Autodesk Inventor part; units mm, degrees
ref_plane "Work Plane1" through (0, 0, -15) normal (0, 0, 1) x (1, 0, 0)
ref_plane "YZ Plane" through (0, 0, 0) normal (1, 0, 0) x (0, 1, 0)
ref_plane "XZ Plane" through (0, 0, 0) normal (0, 1, 0) x (-1, 0, 0)
sketch "Sketch1" plane through (0, 0, 0) normal (0, 0, 1) x (1, 0, 0)
  line L0 (0, 0) -> (25, 0)
  line L1 (25, 0) -> (25, 40)
  line L2 (25, 40) -> (0, 40)
  line L3 (0, 40) -> (0, 0)
  dimension "d1" = 25
  dimension "d2" = 40
  dimension "d3" = 25
extrude "Extrusion1" add sketch "Sketch1" against normal blind 30
sketch "Sketch2" plane through (25, 0, 0) normal (1, 0, 0) x (0, 0, -1)
  line L0 (0, 0) -> (30, 0)
  circle A0 centre (15, 6.56) radius 2.46
extrude "Extrusion2" cut sketch "Sketch2" against normal blind 30
sketch "Sketch3" plane through (0, 0, 0) normal (-1, 0, 0) x (0, 0, 1)
  line L0 (0, 0) -> (-30, 0)
  line L1 (-25.05, 0) -> (-4.95, 0)
  line L2 (-4.95, 0) -> (-4.95, 33.12)
  line L3 (-4.95, 33.12) -> (-25.05, 33.12)
  line L4 (-25.05, 33.12) -> (-25.05, 0)
  dimension "d11" = 20.1
extrude "Extrusion3" cut sketch "Sketch3" against normal blind 20
sketch "Sketch4" plane through (0, 0, 0) normal (0, -1, 0) x (1, 0, 0)
  line L0 (20, -4.95) -> (20, -25.05)
  line L1 (20, -15) -> (25, -15)
  line L2 (25, 0) -> (25, -30)
  line L3 (20, -8.025) -> (25, -8.025)
  line L4 (25, -8.025) -> (25, -21.975)
  line L5 (25, -21.975) -> (20, -21.975)
  line L6 (20, -21.975) -> (20, -8.025)
  line L7 (20, -8.025) -> (25, -21.975) construction
  line L8 (25, -8.025) -> (20, -21.975) construction
  line L9 (25, -12.54) -> (25, -17.46)
  point P0 (0, 0)
  point P1 (22.5, -15)
  dimension "d14" = 13.95
extrude "Extrusion4" add sketch "Sketch4" along normal blind 15
sketch "Sketch5" plane through (20, 0, 0) normal (-1, 0, 0) x (0, 0, 1)
  circle A0 centre (-15, 6.56) radius 2.46
  circle A1 centre (-15, 6.56) radius 4.7025
  circle A2 centre (-15, 6.56) radius 2.46
  circle A3 centre (-15, 6.56) radius 2.46
  point P0 (0, 0)
  dimension "d17" = 9.405
extrude "Extrusion5" cut sketch "Sketch5" against normal blind 2.1
sketch "Sketch6" plane through (25, 0, 0) normal (1, 0, 0) x (0, 0, -1)
  circle A0 centre (15, 6.56) radius 4.7025
  line L0 (15, 6.56) -> (15, 23.56)
  circle A1 centre (15, 23.56) radius 2.46
  point P0 (0, 0)
  dimension "d20" = 17
  dimension "d21" = 4.92
extrude "Extrusion6" cut sketch "Sketch6" against normal blind 10 contours A1
sketch "Sketch7" plane through (20, 0, 0) normal (-1, 0, 0) x (0, 0, 1)
  circle A0 centre (-15, 23.56) radius 2.46
  circle A1 centre (-15, 23.56) radius 4.7025
  point P0 (0, 0)
  dimension "d24" = 9.405
extrude "Extrusion7" cut sketch "Sketch7" against normal blind 2.1
sketch "Sketch9" plane through (25, 0, 0) normal (1, 0, 0) x (0, 0, -1)
  circle A0 centre (15, 6.56) radius 2.46
  circle A1 centre (15, 6.56) radius 2.46
  circle A2 centre (15, 23.56) radius 2.46
  circle A3 centre (15, 23.56) radius 2.46
  line L0 (30, 40) -> (30, 0)
  line L1 (30, 0) -> (30, 40)
  line L2 (30, 40) -> (0, 40)
  line L3 (0, 40) -> (0, 0)
  line L4 (0, 0) -> (8.025, 0)
  line L5 (21.975, 0) -> (21.975, -15)
  line L6 (21.975, -15) -> (8.025, -15)
  line L7 (8.025, -15) -> (8.025, 0)
  line L8 (0, 0) -> (8.025, 0)
  line L9 (21.975, 0) -> (30, 0)
extrude "Extrusion8" add sketch "Sketch9" along normal blind 5
sketch "Sketch10" plane through (0, 40, 0) normal (0, 1, 0) x (1, 0, 0)
  line L0 (0, 30) -> (30, 30)
  line L1 (30, 0) -> (0, 0)
  line L2 (0, 30) -> (30, 30)
  line L3 (30, 30) -> (30, 0)
  line L4 (30, 0) -> (0, 0)
  line L5 (0, 0) -> (0, 30)
extrude "Extrusion9" add sketch "Sketch10" along normal blind 30
sketch "Sketch12" plane through (30, 0, 0) normal (1, 0, 0) x (0, 0, -1)
  circle A0 centre (15, 6.56) radius 2.46
  line L0 (15, 6.56) -> (15, 15.06)
  circle A1 centre (15, 15.06) radius 2.525
  point P0 (0, 0)
  dimension "d31" = 8.5
  dimension "d33" = 5.05
extrude "Extrusion10" cut sketch "Sketch12" against normal blind 30 contours A1
sketch "Sketch15" plane through (0, 0, -25.05) normal (-1, 0, 0) x (0, 0, 1)
  line L0 (0, 33.12) -> (20.1, 33.12)
  line L1 (20.1, 33.12) -> (20.1, 0)
  line L2 (0, 33.12) -> (20.1, 33.12)
  line L3 (20.1, 33.12) -> (20.1, 31.1)
  line L4 (20.1, 31.1) -> (0, 31.1)
  line L5 (0, 31.1) -> (0, 33.12)
  point P0 (25.05, 0)
  dimension "d57" = 2.02
extrude "Extrusion13" add sketch "Sketch15" against normal blind 20
sketch "Sketch17" plane through (0, 0, 0) normal (0, 0, 1) x (1, 0, 0)
  line L0 (0, 70) -> (30, 70)
  line L1 (30, 70) -> (50.0622, 90.0622)
  line L2 (30, 70) -> (80, 70) construction
  line L3 (11.9522, 97.2454) -> (0, 85.2932)
  line L4 (0, 70) -> (0, 85.2932)
  line L5 (0, 70) -> (0, 0)
  line L6 (0, 70) -> (30, 70)
  line L7 (10.923, 112.2849) -> (0, 120.567)
  line L8 (50.0622, 105.3553) -> (50.0622, 120.567)
  line L9 (50.0622, 105.3553) -> (50.0622, 90.0622)
  arc A0 (11.9522, 97.2454) -> (10.923, 112.2849) centre (4.8811, 104.3165) ccw
  line L10 (0, 156.567) -> (30, 156.567)
  line L11 (30, 156.567) -> (50.0622, 120.567)
  line L12 (5, 154.567) -> (0, 156.567)
  line L13 (5, 122.567) -> (0, 120.567)
  line L14 (5, 122.567) -> (10, 138.567)
  line L15 (10, 138.567) -> (5, 154.567)
  dimension "d61" = 45
  dimension "d62" = 32.0271
  dimension "d72" = 10
extrude "Extrusion14" add sketch "Sketch17" against normal blind 30
sketch "Sketch23" plane through (0, 0, 0) normal (0, 0, 1) x (1, 0, 0)
  line L0 (50.0622, 90.0622) -> (30, 70)
  line L1 (30, 70) -> (50.0622, 90.0622)
  line L2 (50.0622, 120.567) -> (50.0622, 90.0622)
  line L3 (50.0622, 90.0622) -> (50.0622, 120.567)
  line L4 (30, 156.567) -> (50.0622, 120.567)
  line L5 (50.0622, 120.567) -> (30, 156.567)
  line L6 (0, 156.567) -> (30, 156.567)
  line L7 (30, 156.567) -> (0, 156.567)
  line L8 (5, 154.567) -> (0, 156.567)
  line L9 (0, 156.567) -> (5, 154.567)
  line L10 (10, 138.567) -> (5, 154.567)
  line L11 (5, 154.567) -> (10, 138.567)
  line L12 (5, 122.567) -> (10, 138.567)
  line L13 (10, 138.567) -> (5, 122.567)
  line L14 (0, 120.567) -> (5, 122.567)
  line L15 (5, 122.567) -> (0, 120.567)
  line L16 (10.923, 112.2849) -> (0, 120.567)
  line L17 (0, 120.567) -> (10.923, 112.2849)
  line L18 (0, 85.2932) -> (11.9522, 97.2454)
  line L19 (11.9522, 97.2454) -> (0, 85.2932)
  line L20 (0, 85.2932) -> (0, 55.2932)
  line L21 (0, 0) -> (0, 85.2932)
  line L22 (0, 55.2932) -> (30, 55.2932)
  line L23 (30, 0) -> (30, 70)
  line L24 (30, 55.2932) -> (30, 70)
  arc A0 (11.9522, 97.2454) -> (10.923, 112.2849) centre (4.8811, 104.3165) ccw
  dimension "d97" = 30
extrude "Extrusion15" add sketch "Sketch23" along normal blind 30
ref_plane "Work Plane1" through (0, 0, -15) normal (0, 0, 1) x (1, 0, 0)
mirror "Mirror1" about plane through (0, 0, -15) normal (0, 0, 1) of "Extrusion15"
properties part number "rec_c_32mm_x_90mm"
Here's how the part is built. I have some questions about the finished solid (model axes, mm). A direction names the side the tool comes from. Give positions to 0.01 mm unless a question says otherwise; leave off trailing zeros. Loops run counter-clockwise (first coordinate to the right, second up) from the corner with the lowest first, then second, coordinate; pieces in that order, holes last. Notation, with made-up numbers: (29.5, 72) -> (88.5, 72) arc R21 ccw to (88.5, 86) -> close; hole circle Ø7 at (74.5, -26.75). An arc over 180 degrees is marked (long way). Answer as a JSON object with one key per item and string values. Group by question number.
Item 1: On a 3-axis mill with a long thin cutter (end or side, diameter ignored), from which of +Z, -Z, +X, -X, +Y, -Y can I reach the whole of each face in a straight line? I mean faces 1 (the flat face through (15, 55.293, -45)), 2 (the flat face through (25, -8, -8.025)), 3 (the flat face through (30, 47, -14)), 4 (the flat face through (7.535, 130.679, -14.37)). Say none if no direction works.
Item 2: Will these pins go through, and if not, where does the flat tip stop? pin 1 (7.5 mm diameter, centred on y = 4, z = -16, fed in from -X); pin 2 (6.5 mm diameter, centred on y = 6.56, z = -15, fed in from -X); pin 3 (4.5 mm diameter, centred on y = 15.06, z = -15, fed in from -X); pin 4 (10 mm diameter, centred on x = 5, y = 18.5, fed in from +Z).
Item 3: Imagine slicing it at D-D on y = 61. Write out the boundary of the cut face in (x, z), then the cut area to 3 significant figures.
Item 4: Imagine slicing it at A-A on y = 23.56. Write out the boundary of the cut face in (x, z), then the cut area to 3 significant figures.
Item 5: Imagine slicing it at B-B on z = 20. Write out the boundary of the cut face in (x, y), then the cut area to 3 significant figures.
Item 6: I need wall thicknesses on L1, parallel to Y at x = 26.75, z = -15 (3 decimals); L2, parallel to Z at x = 27.5, y = 15.06 (3 decimals); L3, parallel to Y at x = 21.05, z = -15 (1 decimal). Which ranges of each line are inside material? Lowest first, please.
Item 7: Imagine slicing it at C-C on z = -15. Give the number of separate pieces and of enclosed holes in the cut face, then the cut area to 3 significant figures.
Item 8: Thinking about a two-plate mould opening in Z: for faces 5 (the flat face through (6.06, 91.353, -14.37)), 6 (the cylindrical face through (25.995, 7.502, -17.272)), 7 (the flat face through (20, 8, -20)), 8 (the flat face through (25, -7, -21.975)), which applies, pulls with the +Z half, pulls with the -Z half, needs draft (parallel to the pull), parting line crosses it, or undercut?
Answer list:
{
 "1": {"face 1": "-Z, +X, -X, -Y", "face 2": "+Z, +X, -X, -Y", "face 3": "+Z, -Z, +X, -Y", "face 4": "+Z, -Z, -X"},
 "2": {"pin 1": "stops at x = 20", "pin 2": "stops at x = 22.1", "pin 3": "passes through", "pin 4": "stops at z = 0"},
 "3": {"outline": "(0, -60) -> (30, -60) -> (30, 30) -> (0, 30) -> close", "area": "2,700 mm2"},
 "4": {"outline": "(0, -30) -> (30, -30) -> (30, -17.46) -> (22.1, -17.46) -> (22.1, -19.7) -> (20, -19.7) -> (20, -25.05) -> (0, -25.05) -> close; (0, -4.95) -> (20, -4.95) -> (20, -10.3) -> (22.1, -10.3) -> (22.1, -12.54) -> (30, -12.54) -> (30, 0) -> (0, 0) -> close", "area": "439 mm2"},
 "5": {"outline": "(0, 55.29) -> (30, 55.29) -> (30, 70) -> (50.06, 90.06) -> (50.06, 120.57) -> (30, 156.57) -> (0, 156.57) -> (5, 154.57) -> (10, 138.57) -> (5, 122.57) -> (0, 120.57) -> (10.92, 112.28) arc R10 cw to (11.95, 97.25) -> (0, 85.29) -> close", "area": "3,640 mm2"},
 "6": {"L1": "y = -15 to 4.1, 9.02 to 12.535, 17.585 to 21.1, 26.02 to 156.567", "L2": "z = -30 to -17.525, -12.475 to 0", "L3": "y = -15 to 1.9, 11.3 to 12.5, 17.6 to 18.9, 28.3 to 156.6"},
 "7": {"separate pieces": "4", "enclosed holes": "0", "area": "4,660 mm2"},
 "8": {"face 5": "needs draft", "face 6": "undercut", "face 7": "undercut", "face 8": "pulls with the -Z half"}
}
